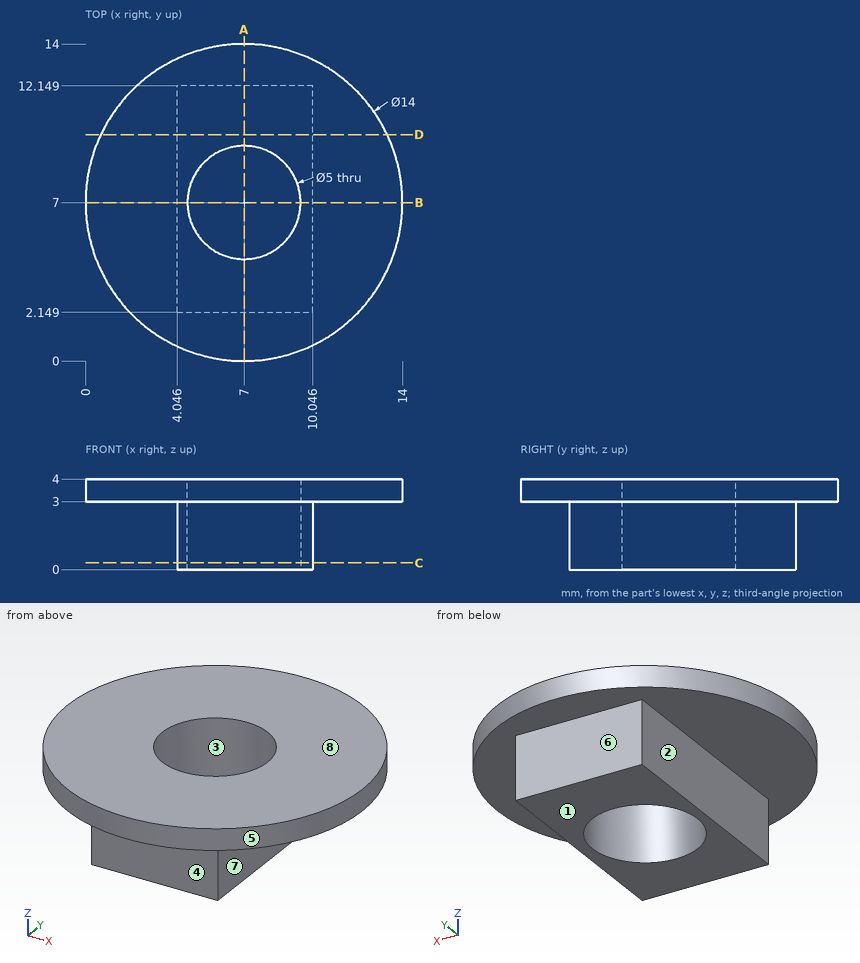
Geometry check sheet. Reference: drawing and pictorial views, mm from the part's lowest x, y, z. A direction names the side the tool comes from. Give positions to 0.01 mm unless a question says otherwise; leave off trailing zeros. Order: outer loops, then holes, each group sorted by start corner. A loop starts at its lowest first (then second) coordinate and runs counter-clockwise, first axis right, second up. Notation, with made-up numbers: M -17.5,10 L 13.5,10 A20 cw 13.5,48 Z; hole C 27,58 d9. An arc over 180 degrees is marked long. Answer in a Markdown table with one row per item.
1) Thickness scan on L1, parallel to Y at x = 7, z = 1.3; L2, parallel to Z at x = 13.25, y = 6.75; L3, parallel to Y at x = 7.5, z = 0.95. Record the ranges inside material, lowest first. Write a range as [from, to].
Filled sheet:
| item | result |
|---|---|
| L1 | y = [2.15, 4.5], [9.5, 12.15] |
| L2 | z = [3, 4] |
| L3 | y = [2.15, 4.55], [9.45, 12.15] |
2) Cross-section at D-D, the plane y = 10. Enter the section's corners in (x, z) (1 decimal).
Filled sheet:
| item | result |
|---|---|
| outline | M 0.7,3 L 4,3 L 4,0 L 10,0 L 10,3 L 13.3,3 L 13.3,4 L 0.7,4 Z |
3) Cross-section at B-B, the plane y = 7. Enter the section's corners in (x, z) (1 decimal).
Filled sheet:
| item | result |
|---|---|
| outline | M 0,3 L 4,3 L 4,0 L 4.5,0 L 4.5,4 L 0,4 Z; M 9.5,0 L 10,0 L 10,3 L 14,3 L 14,4 L 9.5,4 Z |
4) Cross-section at C-C, the plane z = 0.3. Enter the section's corners in (x, y) (1 decimal).
Filled sheet:
| item | result |
|---|---|
| outline | M 4,2.1 L 10,2.1 L 10,12.1 L 4,12.1 Z; hole C 7,7 d5 |
5) Release check for a two-part mould opening along X. For the marked faces 1, 2 and 3 record: +X half, -X half, draft (parallel to the pull), parting line (faces both ways), or undercut.
Filled sheet:
| item | result |
|---|---|
| face 1 | draft |
| face 2 | -X half |
| face 3 | undercut |
6) Access from +Z, -Z, +X, -X, +Y, -Y to the whole of each face (thin tool, end or side, straight path). Record for the marked faces 4, 5, 6, 7 and 8.
Filled sheet:
| item | result |
|---|---|
| face 4 | -Z, +X, -X, -Y |
| face 5 | +Z, -Z |
| face 6 | -Z, +X, -X, +Y |
| face 7 | -Z, +X, +Y, -Y |
| face 8 | +Z, +X, -X, +Y, -Y |
7) Cross-section at A-A, the plane x = 7. Enter the section's corners in (y, z).
Filled sheet:
| item | result |
|---|---|
| outline | M 0,3 L 2.15,3 L 2.15,0 L 4.5,0 L 4.5,4 L 0,4 Z; M 9.5,0 L 12.15,0 L 12.15,3 L 14,3 L 14,4 L 9.5,4 Z |
8) Gauge pin test, flat ends, axial feed: P1, Ø2, axis at x = 4, z = 1.5, coming from the -Y side; P2, Ø1.5, axis at x = 5.5, z = 1, coming from the +Y side; P3, Ø1.5, axis at y = 4.5, z = 2, coming from the +X side. Record the tip position at first contact, or that the pin passes through.
Filled sheet:
| item | result |
|---|---|
| P1 | stops at y = 2.15 |
| P2 | stops at y = 12.15 |
| P3 | stops at x = 10.05 |
